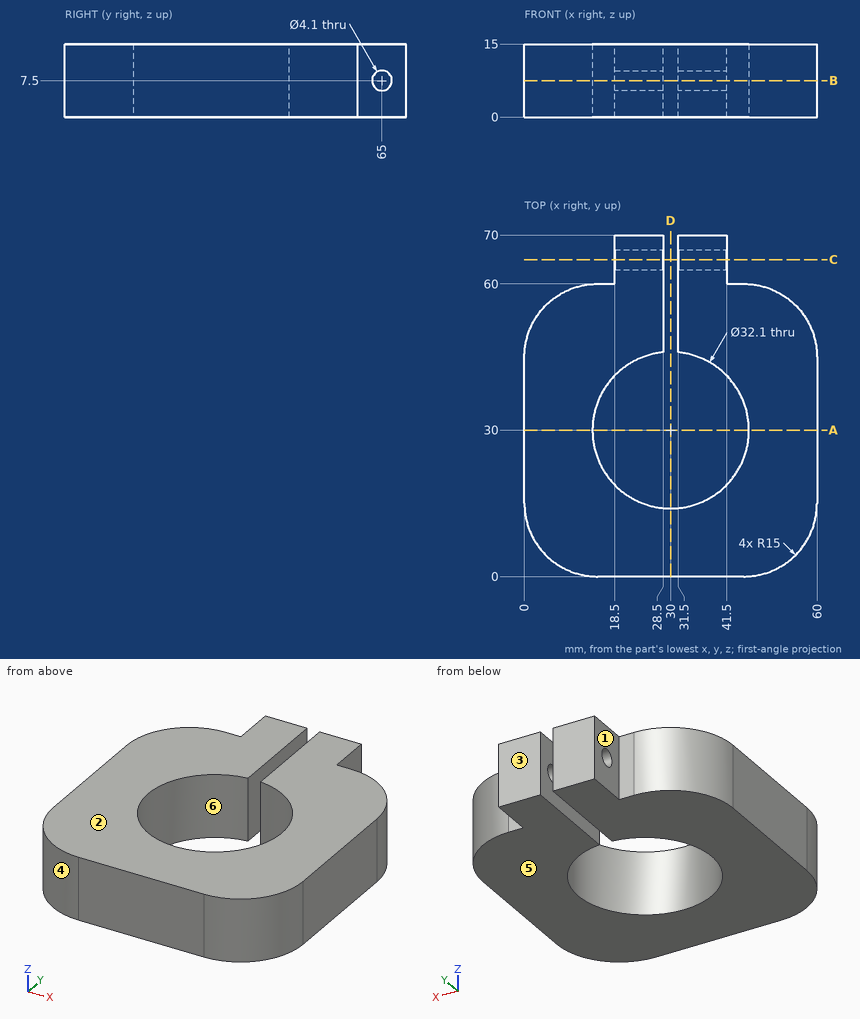
Part print with two shaded views. Sizes in mm from the minimum x, y, z corner. A direction names the side the tool comes from. Give positions to 0.01 mm unless a question says otherwise; leave off trailing zeros. Order: outer loops, then holes, each group sorted by start corner. A loop starts at its lowest first (then second) coordinate and runs counter-clockwise, first axis right, second up.
(1) Saw through at C-C, the plane y = 65. Give the cut face in (x, z), then the cut area to 3 significant figures.
(2) Saw through at A-A, the plane y = 30. Give the cut face in (x, z).
(3) Saw through at B-B, the plane z = 7.5. Give the cut face in (x, y).
(4) Drill centre lines: L1, parallel to Y at x = 34.75, z = 7.5; L2, parallel to X at y = 30, z = 4.5; L3, parallel to Y at x = 19, z = 5.75. Where is each one in solid material? Low to high.
(5) Saw through at D-D, the plane x = 30. Give the cut face in (y, z), then the cut area to 3 significant figures.
(6) Tool access for the marked faces 1 and 2: list every direction of +Z, -Z, +X, -X, +Y, -Y with a clear straight run to the whole face (end or side of a thin tool).
(7) Flat gauge pins, fed straight in: pin 1 (1.8 mm diameter, centred on x = 43.5, z = 6, fed in from +Y); pin 2 (5 mm diameter, centred on y = 58, z = 2, fed in from +X); pin 3 (3 mm diameter, centred on y = 66, z = 7.5, fed in from -X); pin 4 (3.5 mm diameter, centred on y = 65, z = 7.5, fed in from -X). Where does each tip first touch, or does it go through?
(8) Mould opens along Y. For the marked faces 3, 4, 5 and 6 say: released by +Y, released by -Y, zero draft, split by the parting line, or undercut.
Results found:
1. outline: (18.5, 0) - (28.5, 0) - (28.5, 5.45) - (18.5, 5.45) - close; (18.5, 9.55) - (28.5, 9.55) - (28.5, 15) - (18.5, 15) - close; (31.5, 0) - (41.5, 0) - (41.5, 5.45) - (31.5, 5.45) - close; (31.5, 9.55) - (41.5, 9.55) - (41.5, 15) - (31.5, 15) - close
1. area: 218 mm2
2. outline: (0, 0) - (13.95, 0) - (13.95, 15) - (0, 15) - close; (46.05, 0) - (60, 0) - (60, 15) - (46.05, 15) - close
3. outline: (0, 15) arc R15 ccw to (15, 0) - (45, 0) arc R15 ccw to (60, 15) - (60, 45) arc R15 ccw to (45, 60) - (41.5, 60) - (41.5, 62.95) - (31.5, 62.95) - (31.5, 45.98) arc R16.05 cw (long way) to (28.5, 45.98) - (28.5, 62.95) - (18.5, 62.95) - (18.5, 60) - (15, 60) arc R15 ccw to (0, 45) - close; (18.5, 67.05) - (28.5, 67.05) - (28.5, 70) - (18.5, 70) - close; (31.5, 67.05) - (41.5, 67.05) - (41.5, 70) - (31.5, 70) - close
4. L1: y = 0 to 14.67, 45.33 to 62.95, 67.05 to 70
4. L2: x = 0 to 13.95, 46.05 to 60
4. L3: y = 0 to 18.31, 41.69 to 63.93, 66.07 to 70
5. outline: (0, 0) - (13.95, 0) - (13.95, 15) - (0, 15) - close
5. area: 209 mm2
6. face 1: +Z, -Z, -X, +Y
6. face 2: +Z, +X, -X, +Y, -Y
7. pin 1: stops at y = 60
7. pin 2: stops at x = 55.71
7. pin 3: stops at x = 18.5
7. pin 4: passes through
8. face 3: released by +Y
8. face 4: released by -Y
8. face 5: zero draft
8. face 6: undercut
